from build123d import *

# Parameters (mm, degrees)
F0_W     = 50
F0_H     = 15
F0_R     = 2
F1_DEPTH = 3
F2_DEPTH = 6.5
F3_R     = 2.25
F3_R_2   = 2
F4_DEPTH = 2


with BuildPart() as f1:
    # F0 (on Top) → F1 (new body)
    with BuildSketch(Plane.XY):
        with Locations((22.101158835, 0)):
            Rectangle(F0_W, F0_H)
        Circle(F0_R, mode=Mode.SUBTRACT)
        with Locations((16.3239448783, 0)):
            Circle(F0_R, mode=Mode.SUBTRACT)
        with Locations((42.1971863421, 0)):
            Circle(F0_R, mode=Mode.SUBTRACT)
    extrude(amount=F1_DEPTH)

    # F0 (on Top) → F2 (join)
    with BuildSketch(Plane.XY):
        Circle(F0_R)
        with Locations((16.3239448783, 0)):
            Circle(F0_R)
        with Locations((42.1971863421, 0)):
            Circle(F0_R)
    extrude(amount=F2_DEPTH)

    # F3 (on face) → F4 (join)
    with BuildSketch(Plane.XY.offset(6.5)):
        Circle(F3_R)
        Circle(F3_R_2, mode=Mode.SUBTRACT)
        with Locations((16.3239448783, 0)):
            Circle(F3_R)
        with Locations((16.3239448783, 0)):
            Circle(F3_R_2, mode=Mode.SUBTRACT)
        with Locations((42.1971863421, 0)):
            Circle(F3_R)
        with Locations((42.1971863421, 0)):
            Circle(F3_R_2, mode=Mode.SUBTRACT)
        Circle(F3_R_2)
        with Locations((16.3239448783, 0)):
            Circle(F3_R_2)
        with Locations((42.1971863421, 0)):
            Circle(F3_R_2)
    extrude(amount=F4_DEPTH)


solid = f1.part
Here's how the part is built. I have some questions about the finished solid (model axes, mm). A direction names the side the tool comes from. Coordinates: 2 decimals unless noted, no trailing zeros. Write each loop counter-clockwise with the first axis right and the second up, starting at its lowest first coordinate (ties: lowest second). Pieces come first, ordered by that corner, then holes.
1) Which directions (+Z, -Z, +X, -X, +Y, -Y) give clear straight access to the entire face, cutting with the end or side of a thin tool? Please do faces 1 (the face through (-0.29, 2.23, 7.49)), 2 (the face through (40.2, 0.1, 4.7)), 3 (the face through (22, 0, 0)).
Filled in:
face 1: +Z
face 2: none
face 3: -Z, +X, -X, +Y, -Y
2) I'm going to push flat-ended pins straight in: pin 1 (1 mm diameter, centred on y = -2, z = 5, fed in from -X); pin 2 (5 mm diameter, centred on x = 38.5, z = 6.5, fed in from +Y); pin 3 (6 mm diameter, centred on x = 30, y = -5.5, fed in from +Z). Where does each tip first touch, or does it pass through?
Filled in:
pin 1: stops at x = -1.32
pin 2: stops at y = 1.91
pin 3: stops at z = 3
3) If we section it at B-B (x = 0): List the corners of the cut face in (y, z) for me.
Filled in:
outline: (-7.5, 0) - (7.5, 0) - (7.5, 3) - (2, 3) - (2, 6.5) - (2.25, 6.5) - (2.25, 8.5) - (-2.25, 8.5) - (-2.25, 6.5) - (-2, 6.5) - (-2, 3) - (-7.5, 3) - close
4) If we section it at C-C (z = 5.25): List the corners of the cut face in (x, y) for me, plus the area to 3 significant figures.
Filled in:
outline: circle Ø4 at (0, 0); circle Ø4 at (16.32, 0); circle Ø4 at (42.2, 0)
area: 37.7 mm2
5) If we section it at D-D (x = 43.5): List the corners of the cut face in (y, z) for me, plus the area to 3 significant figures.
Filled in:
outline: (-7.5, 0) - (7.5, 0) - (7.5, 3) - (1.52, 3) - (1.52, 6.5) - (1.83, 6.5) - (1.83, 8.5) - (-1.83, 8.5) - (-1.83, 6.5) - (-1.52, 6.5) - (-1.52, 3) - (-7.5, 3) - close
area: 63.0 mm2
6) Thinking about a two-plate mould opening in Z: for faces 4 (the face through (0, -2, 5)), 5 (the face through (42, 0, 8.5)), 6 (the face through (14.076, 0.099, 7.486)), 7 (the face through (14.74, -1.22, 4.73)), which applies, +Z half, -Z half, draft (parallel to the pull), parting line (faces both ways), or undercut?
Filled in:
face 4: undercut
face 5: +Z half
face 6: draft
face 7: undercut
7) If we section it at A-A (y = 0): List the corners of the cut face in (x, z) for me, plus the area to 3 significant figures.
Filled in:
outline: (-2.9, 0) - (47.1, 0) - (47.1, 3) - (44.2, 3) - (44.2, 6.5) - (44.45, 6.5) - (44.45, 8.5) - (39.95, 8.5) - (39.95, 6.5) - (40.2, 6.5) - (40.2, 3) - (18.32, 3) - (18.32, 6.5) - (18.57, 6.5) - (18.57, 8.5) - (14.07, 8.5) - (14.07, 6.5) - (14.32, 6.5) - (14.32, 3) - (2, 3) - (2, 6.5) - (2.25, 6.5) - (2.25, 8.5) - (-2.25, 8.5) - (-2.25, 6.5) - (-2, 6.5) - (-2, 3) - (-2.9, 3) - close
area: 219 mm2
8) If I drill on line 1 (X direction, y = -1.75, z = 8); line 2 (X direction, y = 1.5, z = 3.5); line 3 (Z direction, x = 7, y = 3.5), over which ranges is the centre line in solid material (lowest first)?
Filled in:
line 1: x = -1.41 to 1.41, 14.91 to 17.74, 40.78 to 43.61
line 2: x = -1.32 to 1.32, 15 to 17.65, 40.87 to 43.52
line 3: z = 0 to 3
